Read the model definition and answer for the solid it produces. Units are mm, in the model's axes. Face numbers are marked on the shaded views. A direction names the side the tool comes from. Round coordinates to 2 decimals unless told otherwise and drop trailing zeros. Write each loop counter-clockwise with the first axis right and the second up, starting at its lowest first coordinate (ties: lowest second). Pieces come first, ordered by that corner, then holes. Notation, with made-up numbers: (58.5, 84) -> (78.5, 84) arc R15 cw to (78.5, 93) -> close; hole circle Ø6 at (32.25, -35.75). An arc over 180 degrees is marked (long way). Return JSON: item names as keys, results as strings. Group by question number.
(1) Given pin 1 (1.5 mm diameter, centred on y = 4, z = 3.5, fed in from -X), flat-ended and moving along its own axis, determine where the tip first touches the part or whether it passes through.
(2) For the marked faces 1 and 2, determine the directions among +Z, -Z, +X, -X, +Y, -Y from which every point of the face is accessible in a straight line to the end or side of a thin tool.
(3) A cutting plane is placed at B-B on z = 2.45. State how many separate pieces and enclosed holes the cut face has, then the cut area to 3 significant figures.
(4) A cutting plane is placed at A-A on x = -4.5. Give the vertices of the cut face in (y, z), then the cut area to 3 significant figures.
(5) Straight lines are drawn through the part: line 1 (X direction, y = 1.25, z = 0.8); line 2 (Y direction, x = -11, z = 2.15); line 3 (X direction, y = -0.5, z = 4.3). For each, find the intervals that lie inside material, in ascending order.
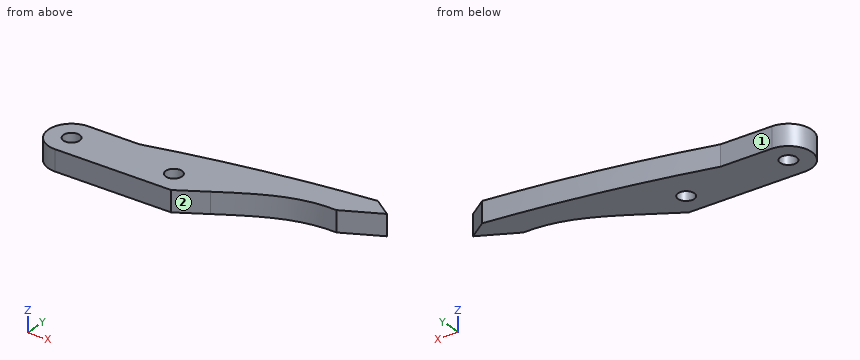
```python
from build123d import *

# Parameters (mm, degrees)
SKETCH2_R           = 5
SKETCH2_R_2         = 1.75
BOSS_EXTRUDE1_DEPTH = 4.5
BOSS_EXTRUDE2_START = -4.5
BOSS_EXTRUDE2_DEPTH = 4.5


with BuildPart() as part:
    # Sketch2 → Boss-Extrude1 (new body)
    # profile 1 of 3: a face of its own
    with BuildSketch(Plane.XY):
        with Locations((-11, 0)):
            Circle(SKETCH2_R)
        with Locations((-11, 0)):
            Circle(SKETCH2_R_2, mode=Mode.SUBTRACT)
    # profile 2 of 3: a face of its own
    with BuildSketch(Plane.XY):
        with Locations((11, 0)):
            Circle(SKETCH2_R)
        with Locations((11, 0)):
            Circle(SKETCH2_R_2, mode=Mode.SUBTRACT)
    # profile 3 of 3: a face of its own
    with BuildSketch(Plane.XY):
        with BuildLine():
            Line((11.000000016, 5), (-11, 5))
            ThreePointArc((-11, 5), (-7.464466094, 3.535533906), (-6, 0))
            ThreePointArc((-6, 0), (-7.464466094, -3.535533906), (-11, -5))
            Line((-11, -5), (11, -5))
            ThreePointArc((11, -5), (6, 8e-09), (11.000000016, 5))
        make_face()
    extrude(amount=BOSS_EXTRUDE1_DEPTH)

    # Sketch3 → Boss-Extrude2 (add)
    with BuildSketch(Plane.XY.offset(4.5).offset(BOSS_EXTRUDE2_START)):
        with BuildLine():
            Line((49.688970331, 10.03), (45.688970331, 12.87))
            add(Edge.make_bspline(
                [(0, 5), (22.564264041, 10.590261298), (45.688970331, 12.87)],
                knots=[0, 0, 0, 1, 1, 1], degree=2))
            Line((0, 5), (11, 5))
            ThreePointArc((11, 5), (16, 0), (11, -5))
            Line((11, -5), (13.99, -5))
            Line((13.99, -5), (19.942130619, -1.48))
            add(Edge.make_bspline(
                [(41.688970331, 6), (33.285520943, 6.459476071), (26.91839773, 2.645658828), (19.942130619, -1.48)],
                knots=[0, 0, 0, 0, 1, 1, 1, 1], degree=3))
            Line((41.688970331, 6), (49.688970331, 10.03))
        make_face()
    extrude(amount=BOSS_EXTRUDE2_DEPTH)


solid = part.part
```
Checks:
{
 "1": {"pin 1": "stops at x = -14.8"},
 "2": {"face 1": "+Z, -Z, -X, +Y", "face 2": "+Z, -Z, +X, -Y"},
 "3": {"separate pieces": "1", "enclosed holes": "2", "area": "559 mm^2"},
 "4": {"outline": "(-5, 0) -> (5, 0) -> (5, 4.5) -> (-5, 4.5) -> close", "area": "45.0 mm^2"},
 "5": {"line 1": "x = -15.84 to -12.22, -9.78 to 9.78, 12.22 to 24.66", "line 2": "y = -5 to -1.75, 1.75 to 5", "line 3": "x = -15.97 to -12.68, -9.32 to 9.32, 12.68 to 21.6"}
}
